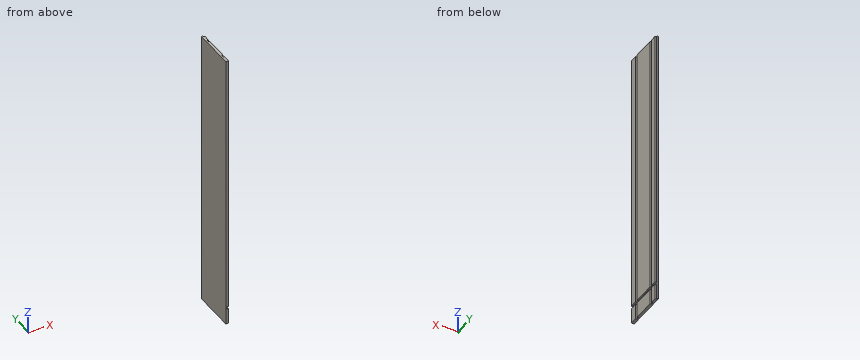
```python
from build123d import *

# Parameters (mm, degrees)
F0_W     = 298.45
F0_H     = 1965.325
F1_DEPTH = 19.05
F2_W     = 298.45
F2_H     = 19.05
F3_DEPTH = 9.525
F4_W     = 19.05
F4_H     = 1965.325
F5_DEPTH = 9.525
F6_W     = 9.525
F6_H     = 9.525
F7_DEPTH = 1965.326


with BuildPart() as f1:
    # F0 (on Right) → F1 (new body)
    with BuildSketch(Plane.YZ):
        Rectangle(F0_W, F0_H)
    extrude(amount=F1_DEPTH)

    # F2 (on face) → F3 (cut)
    with BuildSketch(Plane.YZ.offset(19.05)):
        with Locations((0, -865.1875)):
            Rectangle(F2_W, F2_H)
    extrude(amount=-F3_DEPTH, mode=Mode.SUBTRACT)

    # F4 (on face) → F5 (cut)
    with BuildSketch(Plane.YZ.offset(19.05)):
        with Locations((-88.9, 0)):
            Rectangle(F4_W, F4_H)
        with Locations((88.9, 0)):
            Rectangle(F4_W, F4_H)
    extrude(amount=-F5_DEPTH, mode=Mode.SUBTRACT)

    # F6 (on face) → F7 (cut, through all)
    with BuildSketch(Plane(origin=(0, 0, -982.6625), x_dir=(1, 0, 0), z_dir=(0, 0, -1))):
        with Locations((14.2875, -144.4625)):
            Rectangle(F6_W, F6_H)
    extrude(amount=-F7_DEPTH, mode=Mode.SUBTRACT)


solid = f1.part
```
Read the model definition and answer for the solid it produces. Units are mm, in the model's axes. Give positions to 0.01 mm unless a question says otherwise; leave off trailing zeros. Order: outer loops, then holes, each group sorted by start corner. A loop starts at its lowest first (then second) coordinate and runs counter-clockwise, first axis right, second up.
(1) Find section B-B (z = -111.5). Give the vertices of the cut face in (x, y) (3 decimals).
(2) Find section A-A (x = 14). Give the vertices of the cut face in (y, z) (1 decimal).
(3) Given pin 1 (7.5 mm diameter, centred on x = 13.5, z = -299.5, fed in from +Y); pin 2 (7.5 mm diameter, centred on x = 13, z = -309.5, fed in from +Y) (3 decimals), each flat-ended and moving along its own axis, determine where each tip first touches the part or whether it passes through.
(4) Straight lines are drawn through the part: L1, parallel to Y at x = 17.25, z = 485 (3 decimals); L2, parallel to Z at x = 11.5, y = -132; L3, parallel to X at y = -90, z = -873.5 (3 decimals). For each, find the intervals that lie inside material, in ascending order.
Result sheet:
1. outline: (0, -149.225) - (19.05, -149.225) - (19.05, -98.425) - (9.525, -98.425) - (9.525, -79.375) - (19.05, -79.375) - (19.05, 79.375) - (9.525, 79.375) - (9.525, 98.425) - (19.05, 98.425) - (19.05, 139.7) - (9.525, 139.7) - (9.525, 149.225) - (0, 149.225) - close
2. outline: (-149.2, -982.7) - (-98.4, -982.7) - (-98.4, -874.7) - (-149.2, -874.7) - close; (-149.2, -855.7) - (-98.4, -855.7) - (-98.4, 982.7) - (-149.2, 982.7) - close; (-79.4, -982.7) - (79.4, -982.7) - (79.4, -874.7) - (-79.4, -874.7) - close; (-79.4, -855.7) - (79.4, -855.7) - (79.4, 982.7) - (-79.4, 982.7) - close; (98.4, -982.7) - (139.7, -982.7) - (139.7, -874.7) - (98.4, -874.7) - close; (98.4, -855.7) - (139.7, -855.7) - (139.7, 982.7) - (98.4, 982.7) - close
3. pin 1: stops at y = 139.7
3. pin 2: stops at y = 149.225
4. L1: y = -149.225 to -98.425, -79.375 to 79.375, 98.425 to 139.7
4. L2: z = -982.66 to -874.71, -855.66 to 982.66
4. L3: x = 0 to 9.525
